For this review, take the finished solid that the model builds, in its own axes (mm). A direction names the side the tool comes from. Round coordinates to 2 decimals unless told otherwise and drop trailing zeros. Order: outer loops, then holes, each group sorted by start corner. A loop starts at its lowest first (then second) coordinate and runs counter-clockwise, first axis right, second up. Notation, with made-up numbers: M 68.25,58 L 124.25,58 A7 ccw 124.25,70 Z; hole C 20.5,8 d9. An arc over 180 degrees is marked long. Answer in a Markdown table with one row per item. Add a question column.
```python
from build123d import *

# Parameters (mm, degrees)
SKETCH1_W           = 30
SKETCH1_H           = 30
BOSS_EXTRUDE1_DEPTH = 2
SKETCH2_W           = 5
SKETCH2_H           = 24
BOSS_EXTRUDE2_DEPTH = 10
SKETCH3_W           = 5
SKETCH3_H           = 5
SKETCH3_H_2         = 8
CUT_EXTRUDE1_DEPTH  = 8
SKETCH4_R           = 2.25
CUT_EXTRUDE2_DEPTH  = 10


with BuildPart() as part:
    # Sketch1 → Boss-Extrude1 (new body)
    with BuildSketch(Plane(origin=(0, 0, 0), x_dir=(1, 0, 0), z_dir=(0, 1, 0))):
        with Locations((15, 15)):
            Rectangle(SKETCH1_W, SKETCH1_H)
    extrude(amount=BOSS_EXTRUDE1_DEPTH)

    # Sketch2 → Boss-Extrude2 (add)
    with BuildSketch(Plane(origin=(0, 2, 0), x_dir=(1, 0, 0), z_dir=(0, 1, 0))):
        with Locations((4, 15)):
            Rectangle(SKETCH2_W, SKETCH2_H)
    extrude(amount=BOSS_EXTRUDE2_DEPTH)

    # Sketch3 → Cut-Extrude1 (cut)
    with BuildSketch(Plane(origin=(0, 12, 0), x_dir=(1, 0, 0), z_dir=(0, 1, 0))):
        with Locations((4, 24.5)):
            Rectangle(SKETCH3_W, SKETCH3_H)
        with Locations((4, 5.5)):
            Rectangle(SKETCH3_W, SKETCH3_H)
        with Locations((4, 15)):
            Rectangle(SKETCH3_W, SKETCH3_H_2)
    extrude(amount=-CUT_EXTRUDE1_DEPTH, mode=Mode.SUBTRACT)

    # Sketch4 → Cut-Extrude2 (cut)
    with BuildSketch(Plane.XZ):
        with Locations(Location((25.390935128, -5, 0), (0, 0, 270))):
            Circle(SKETCH4_R)
        with Locations(Location((25.390935128, -25, 0), (0, 0, 270))):
            Circle(SKETCH4_R)
    extrude(amount=-CUT_EXTRUDE2_DEPTH, mode=Mode.SUBTRACT)


solid = part.part
```
1. Consider section B-B on z = -25. Write out the cut boundary in (x, y).
2. Consider section A-A on y = 8.25. Write out the cut boundary in (x, z), plus the area to 3 significant figures.
3. To check wall thickness, follow probe 1 along Z at (x, y) = (4, 9.5); probe 2 along X at (y, z) = (1.65, -5); probe 3 along Y at (x, z) = (22, -1.75). State the ranges of each line that lie inside material, in increasing order. Write a range as [from, to].
4. Consider section D-D on x = 22.5. Write out the cut boundary in (y, z), plus the area to 3 significant figures.
5. For faces 1 (the flat face through (4, 8, -8)), 2 (the flat face through (1.5, 3.6, -14.8)), 3 (the flat face through (4, 4, -25)), 4 (the flat face through (4, 8, -19)), list the 3-axis set-ups (+Z, -Z, +X, -X, +Y, -Y) from which the entire face can be reached by the end or side of a thin tool; tool diameter is ignored.
6. The part is to be moulded in two halves that separate along X. For faces 5 (the flat face through (15, 2, -15)), 6 (the flat face through (6.5, 3.6, -14.8)), 7 (the cylindrical face through (27.622, 0.986, -4.707)), say which applies: pulls with the +X half, pulls with the -X half, needs draft (parallel to the pull), parting line crosses it, or undercut.
7. Clearance check with flat-ended pins moving along their axes: pin 1 Ø4 at (x, z) = (13, -26.5) entering from +Y; pin 2 Ø4 at (x, z) = (5, -25.5) entering from +Y; pin 3 Ø5.5 at (x, y) = (5, 8) entering from +Z; pin 4 Ø1.6 at (x, y) = (5, 2.5) entering from +Z. State where each tip first meets the part, or that it passes through.
8. Consider section C-C on z = -20.25. Write out the cut boundary in (x, y), plus the area to 3 significant figures.
Solved:
| question | item | result |
|---|---|---|
| 1 | outline | M 0,0 L 23.14,0 L 23.14,2 L 6.5,2 L 6.5,4 L 1.5,4 L 1.5,2 L 0,2 Z; M 27.64,0 L 30,0 L 30,2 L 27.64,2 Z |
| 2 | outline | M 1.5,-22 L 6.5,-22 L 6.5,-19 L 1.5,-19 Z; M 1.5,-11 L 6.5,-11 L 6.5,-8 L 1.5,-8 Z |
| 2 | area | 30.0 mm^2 |
| 3 | probe 1 | z = [-22, -19], [-11, -8] |
| 3 | probe 2 | x = [0, 23.14], [27.64, 30] |
| 3 | probe 3 | y = [0, 2] |
| 4 | outline | M 0,-30 L 2,-30 L 2,0 L 0,0 Z |
| 4 | area | 60.0 mm^2 |
| 5 | face 1 | +Z, +X, -X, +Y |
| 5 | face 2 | +Z, -Z, -X, +Y |
| 5 | face 3 | -Z, +X, -X, +Y |
| 5 | face 4 | +X, -X, +Y |
| 6 | face 5 | needs draft |
| 6 | face 6 | pulls with the +X half |
| 6 | face 7 | undercut |
| 7 | pin 1 | stops at y = 2 |
| 7 | pin 2 | stops at y = 4 |
| 7 | pin 3 | stops at z = -8 |
| 7 | pin 4 | stops at z = 0 |
| 8 | outline | M 0,0 L 30,0 L 30,2 L 6.5,2 L 6.5,12 L 1.5,12 L 1.5,2 L 0,2 Z |
| 8 | area | 110 mm^2 |
